Read the model definition and answer for the solid it produces. Units are mm, in the model's axes. A direction names the side the tool comes from. Coordinates: 2 decimals unless noted, no trailing zeros. Write each loop counter-clockwise with the first axis right and the second up, starting at its lowest first coordinate (ties: lowest second). Pieces come first, ordered by that corner, then holes. Notation, with made-up numbers: (47, 37) - (96, 37) arc R37 ccw to (96, 75) - close; hole circle Ø11 at (-37, 75.5). An arc over 180 degrees is marked (long way). Use a Markdown table: item, result.
from build123d import *

# Parameters (mm, degrees)
BOSS_EXTRUDE1_DEPTH = 203.2
CUT_EXTRUDE1_DEPTH  = 7.112


with BuildPart() as part:
    # end-profile → Boss-Extrude1 (new body)
    with BuildSketch(Plane.XY):
        Polygon((0, 0), (-7.751918639, 0), (-18.867713308, 15.875), (-11.115794669, 15.875), align=None)
    extrude(amount=BOSS_EXTRUDE1_DEPTH)

    # Sketch4 → Cut-Extrude1 (cut)
    with BuildSketch(Plane(origin=(-18.867713308, 0, 0), x_dir=(0, 0, -1), z_dir=(1, 0, 0))):
        with BuildLine():
            Line((-180.141175267, 7.9375), (-180.141175267, 0))
            Line((-180.141175267, 0), (-173.366995267, 0))
            Line((-173.366995267, 0), (-173.366995267, 7.9375))
            ThreePointArc((-173.366995267, 7.9375), (-176.754085267, 11.32459), (-180.141175267, 7.9375))
        make_face()
        with BuildLine():
            Line((-142.041175267, 7.9375), (-142.041175267, 0))
            Line((-142.041175267, 0), (-135.266995267, 0))
            Line((-135.266995267, 0), (-135.266995267, 7.9375))
            ThreePointArc((-135.266995267, 7.9375), (-138.654085267, 11.32459), (-142.041175267, 7.9375))
        make_face()
        with BuildLine():
            Line((-103.941175267, 7.9375), (-103.941175267, 0))
            Line((-103.941175267, 0), (-97.166995267, 0))
            Line((-97.166995267, 0), (-97.166995267, 7.9375))
            ThreePointArc((-97.166995267, 7.9375), (-100.554085267, 11.32459), (-103.941175267, 7.9375))
        make_face()
        with BuildLine():
            Line((-65.841175267, 7.9375), (-65.841175267, 0))
            Line((-65.841175267, 0), (-59.066995267, 0))
            Line((-59.066995267, 0), (-59.066995267, 7.9375))
            ThreePointArc((-59.066995267, 7.9375), (-62.454085267, 11.32459), (-65.841175267, 7.9375))
        make_face()
        with BuildLine():
            Line((-27.741175267, 7.9375), (-27.741175267, 0))
            Line((-27.741175267, 0), (-20.966995267, 0))
            Line((-20.966995267, 0), (-20.966995267, 7.9375))
            ThreePointArc((-20.966995267, 7.9375), (-24.354085267, 11.32459), (-27.741175267, 7.9375))
        make_face()
    extrude(amount=CUT_EXTRUDE1_DEPTH, mode=Mode.SUBTRACT)


solid = part.part
(1) A cutting plane is placed at B-B, the plane x = -3.5. Write down the section's boundary in (y, z).
Report:
| item | result |
|---|---|
| outline | (0, 0) - (5, 0) - (5, 203.2) - (0, 203.2) - close |
(2) Each of these flat-tipped pins is pushed along its axis until it touches: P1, Ø6, axis at y = 4, z = 114.5, coming from the -X side; P2, Ø3, axis at y = 7.5, z = 138, coming from the -X side; P3, Ø10, axis at x = -2.5, z = 115.5, coming from the +Y side. Where does it stop, or does it pass through?
Report:
| item | result |
|---|---|
| P1 | stops at x = -12.65 |
| P2 | stops at x = -11.76 |
| P3 | stops at y = 10.71 |
(3) A cutting plane is placed at A-A, the plane z = 62. Write down the section's boundary in (x, y) (3 decimals), and give its area (3 significant figures).
Report:
| item | result |
|---|---|
| outline | (-18.868, 15.875) - (-15.66, 11.294) - (-11.756, 11.294) - (-11.756, 5.718) - (-7.752, 0) - (0, 0) - (-11.116, 15.875) - close |
| area | 112 mm² |
(4) For faces 1 (the flat face through (-11.756, 8, 63)), 2 (the flat face through (-4, 0, 100)), determine the directions among +Z, -Z, +X, -X, +Y, -Y from which every point of the face is accessible in a straight line to the end or side of a thin tool.
Report:
| item | result |
|---|---|
| face 1 | -X, -Y |
| face 2 | +Z, -Z, +X, -X, -Y |
(5) A cutting plane is placed at C-C, the plane y = 13. Write down the section's boundary in (x, z), and give its area (3 significant figures).
Report:
| item | result |
|---|---|
| outline | (-16.85, 0) - (-9.1, 0) - (-9.1, 203.2) - (-16.85, 203.2) - close |
| area | 1,580 mm² |
(6) The mould has two halves that part along Z. Classify faces 3 (the cylindrical face through (-13.31, 11.324, 176.68)), 4 (the flat face through (-10.762, 4.299, 100.178)), 5 (the flat face through (-9, 8, 0)): pulls with the +Z half, pulls with the -Z half, needs draft (parallel to the pull), parting line crosses it, or undercut.
Report:
| item | result |
|---|---|
| face 3 | undercut |
| face 4 | needs draft |
| face 5 | pulls with the -Z half |
(7) Straight lines are drawn through the part: L1, parallel to Y at x = -6.25, z = 154; L2, parallel to Y at x = -13, z = 183 (3 decimals); L3, parallel to X at y = 3, z = 16. For each, find the intervals that lie inside material, in ascending order.
Report:
| item | result |
|---|---|
| L1 | y = 0 to 8.93 |
| L2 | y = 7.495 to 15.875 |
| L3 | x = -9.85 to -2.1 |
